Source: CAD feature listing. Evaluate the final solid. Frame: model axes, mm. Face numbers are marked on the shaded views. A direction names the side the tool comes from. Coordinates: 2 decimals unless noted, no trailing zeros. Order: outer loops, then holes, each group sorted by start corner. A loop starts at its lowest first (then second) coordinate and runs counter-clockwise, first axis right, second up.
```python
from build123d import *

# Parameters (mm, degrees)
CROQUIS1_W              = 70
CROQUIS1_H              = 50
SALIENTE_EXTRUIR1_DEPTH = 30
CROQUIS3_W              = 50
CROQUIS3_H              = 10
CORTAR_EXTRUIR1_DEPTH   = 67
CROQUIS4_R              = 10
CORTAR_EXTRUIR2_DEPTH   = 10


with BuildPart() as part:
    # Croquis1 → Saliente-Extruir1 (new body)
    with BuildSketch(Plane.XY):
        with Locations((35, 25)):
            Rectangle(CROQUIS1_W, CROQUIS1_H)
    extrude(amount=SALIENTE_EXTRUIR1_DEPTH)

    # Croquis3 → Cortar-Extruir1 (cut)
    with BuildSketch(Plane(origin=(0, 0, 0), x_dir=(1, 0, 0), z_dir=(0, 1, 0))):
        with Locations((35, -15)):
            Rectangle(CROQUIS3_W, CROQUIS3_H)
    extrude(amount=CORTAR_EXTRUIR1_DEPTH, mode=Mode.SUBTRACT)

    # Croquis4 → Cortar-Extruir2 (cut)
    with BuildSketch(Plane.XY.offset(30)):
        with Locations((35, 25)):
            Circle(CROQUIS4_R)
    extrude(amount=-CORTAR_EXTRUIR2_DEPTH, mode=Mode.SUBTRACT)


solid = part.part
```
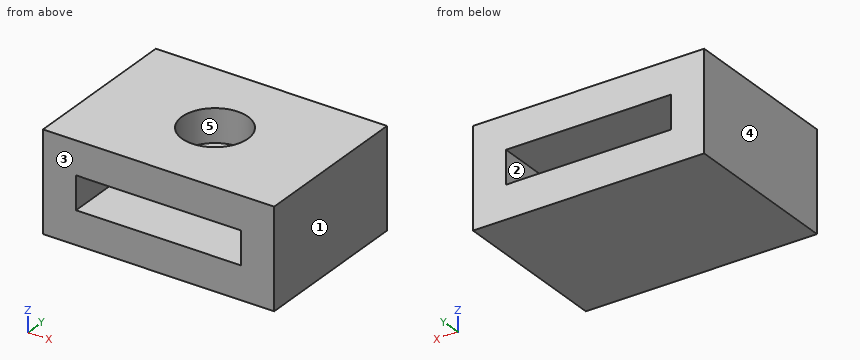
1. Section query B-B on z = 22.25. Return loops of the section in (x, y), plus the area to 3 significant figures.
Findings:
outline: (0, 0) - (70, 0) - (70, 50) - (0, 50) - close; hole circle Ø20 at (35, 25)
area: 3,190 mm2
2. Draft query along X for the marked faces 3, 4 and 5. Return one class per face: released by +X, released by -X, zero draft, split by the parting line, or undercut.
Findings:
face 3: zero draft
face 4: released by -X
face 5: undercut
3. Access query for the marked faces 1 and 2. Directions: +Z, -Z, +X, -X, +Y, -Y. A direction counts if a zero-diameter tool reaches every point of the face in a straight line with its end or side. Return the directions, or none.
Findings:
face 1: +Z, -Z, +X, +Y, -Y
face 2: +Y, -Y
4. Ray query, line 1 (Y direction, x = 35, z = 25.25); line 2 (Z direction, x = 41.5, y = 41); line 3 (X direction, y = 18, z = 13.25). Return the intervals inside material, ascending.
Findings:
line 1: y = 0 to 15, 35 to 50
line 2: z = 0 to 10, 20 to 30
line 3: x = 0 to 10, 60 to 70
5. Section query A-A on x = 35. Return loops of the section in (y, z), plus the area to 3 significant figures.
Findings:
outline: (0, 0) - (50, 0) - (50, 10) - (0, 10) - close; (0, 20) - (15, 20) - (15, 30) - (0, 30) - close; (35, 20) - (50, 20) - (50, 30) - (35, 30) - close
area: 800 mm2
6. Section query D-D on x = 19. Return loops of the section in (y, z).
Findings:
outline: (0, 0) - (50, 0) - (50, 10) - (0, 10) - close; (0, 20) - (50, 20) - (50, 30) - (0, 30) - close
7. Section query C-C on y = 13.5. Return loops of the section in (x, z).
Findings:
outline: (0, 0) - (70, 0) - (70, 30) - (0, 30) - close; hole (10, 10) - (60, 10) - (60, 20) - (10, 20) - close
